Could you check a few things on this model? Use its own coordinates, in mm. Give positions to 0.01 mm unless a question says otherwise; leave off trailing zeros. Order: outer loops, then holes, each group sorted by start corner. A loop starts at its lowest first (then second) coordinate and runs counter-clockwise, first axis right, second up.
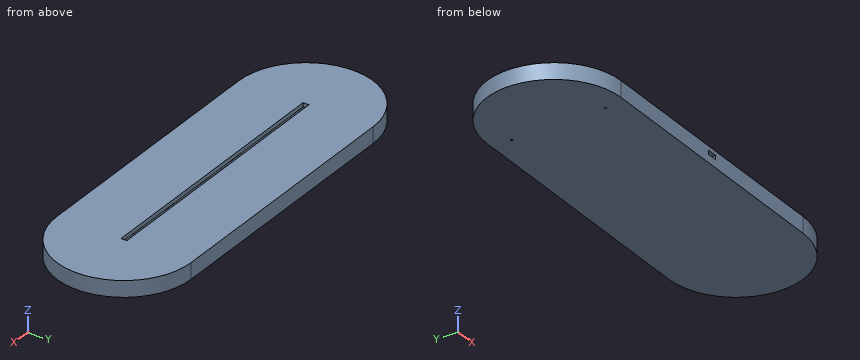
from build123d import *

# Parameters (mm, degrees)
PAD_DEPTH       = 3
PAD001_DEPTH    = 3
SKETCH002_W     = 209.08447
SKETCH002_H     = 4.18
PAD002_DEPTH    = 3
SKETCH003_W     = 26.3
SKETCH003_H     = 34.2
POCKET_DEPTH    = 3
SKETCH004_W     = 18
SKETCH004_H     = 25
POCKET001_DEPTH = 3
SKETCH005_W     = 14
SKETCH005_H     = 5
POCKET002_DEPTH = 6
SKETCH006_W     = 14
SKETCH006_H     = 3
POCKET003_DEPTH = 3
SKETCH007_W     = 8
SKETCH007_H     = 3
POCKET004_DEPTH = 3
SKETCH008_W     = 200
SKETCH008_H     = 4.4
PAD003_DEPTH    = 3
SKETCH009_R     = 0.8
POCKET005_DEPTH = 9


with BuildPart() as part:
    # Sketch → Pad (new body)
    with BuildSketch(Plane.XY):
        with BuildLine():
            ThreePointArc((-100, 50), (-150, 0), (-100, -50))
            Line((-100, -50), (100, -50))
            ThreePointArc((100, -50), (150, 0), (100, 50))
            Line((-100, 50), (100, 50))
        make_face()
    extrude(amount=PAD_DEPTH)

    # Sketch001 (on Face6 of Pad) → Pad001 (join)
    with BuildSketch(Plane.XY.offset(3)):
        with BuildLine():
            ThreePointArc((-100, 50), (-150, 0), (-100, -50))
            Line((-100, -50), (100, -50))
            ThreePointArc((100, -50), (150, 0), (100, 50))
            Line((-100, 50), (100, 50))
        make_face()
        with BuildLine():
            ThreePointArc((-100, 5), (-105, 0), (-100, -5))
            Line((-100, -5), (100, -5))
            ThreePointArc((100, -5), (105, 0), (100, 5))
            Line((-100, 5), (100, 5))
        make_face(mode=Mode.SUBTRACT)
    extrude(amount=PAD001_DEPTH)

    # Sketch002 (on Face9 of Pad001) → Pad002 (join)
    with BuildSketch(Plane.XY.offset(6)):
        with BuildLine():
            ThreePointArc((-100, 50), (-150, 0), (-100, -50))
            Line((-100, -50), (100, -50))
            ThreePointArc((100, -50), (150, 0), (100, 50))
            Line((-100, 50), (100, 50))
        make_face()
        Rectangle(SKETCH002_W, SKETCH002_H, mode=Mode.SUBTRACT)
    extrude(amount=PAD002_DEPTH)

    # Sketch003 (on Face13 of Pad002) → Pocket (cut)
    with BuildSketch(Plane.XY.offset(9)):
        with Locations((0, -29.9)):
            Rectangle(SKETCH003_W, SKETCH003_H)
    extrude(amount=-POCKET_DEPTH, mode=Mode.SUBTRACT)

    # Sketch004 (on Face27 of Pocket) → Pocket001 (cut)
    with BuildSketch(Plane.XY.offset(6)):
        with Locations((0, -25.3)):
            Rectangle(SKETCH004_W, SKETCH004_H)
    extrude(amount=-POCKET001_DEPTH, mode=Mode.SUBTRACT)

    # Sketch005 (on Face13 of Pocket001) → Pocket002 (cut)
    with BuildSketch(Plane.XY.offset(9)):
        with Locations((0, -10.3)):
            Rectangle(SKETCH005_W, SKETCH005_H)
    extrude(amount=-POCKET002_DEPTH, mode=Mode.SUBTRACT)

    # Sketch006 (on Face23 of Pocket002) → Pocket003 (cut)
    with BuildSketch(Plane.XZ.offset(7.8)):
        with Locations((0, 4.5)):
            Rectangle(SKETCH006_W, SKETCH006_H)
    extrude(amount=-POCKET003_DEPTH, mode=Mode.SUBTRACT)

    # Sketch007 (on Face13 of Pocket003) → Pocket004 (cut)
    with BuildSketch(Plane.XY.offset(9)):
        with Locations((0, -48.5)):
            Rectangle(SKETCH007_W, SKETCH007_H)
    extrude(amount=-POCKET004_DEPTH, mode=Mode.SUBTRACT)

    # Sketch008 (on Face15 of Pocket004) → Pad003 (join)
    with BuildSketch(Plane.XY.offset(9)):
        with BuildLine():
            ThreePointArc((-100, 50), (-150, 0), (-100, -50))
            Line((-100, -50), (100, -50))
            ThreePointArc((100, -50), (150, 0), (100, 50))
            Line((-100, 50), (100, 50))
        make_face()
        Rectangle(SKETCH008_W, SKETCH008_H, mode=Mode.SUBTRACT)
    extrude(amount=PAD003_DEPTH)

    # Sketch009 (on Face4 of Pad003) → Pocket005 (cut)
    with BuildSketch(Plane(origin=(0, 0, 0), x_dir=(1, 0, 0), z_dir=(0, 0, -1))):
        with Locations((-95, 35)):
            Circle(SKETCH009_R)
        with Locations((-95, -35)):
            Circle(SKETCH009_R)
    extrude(amount=-POCKET005_DEPTH, mode=Mode.SUBTRACT)


solid = part.part
Item 1: Imagine slicing it at A-A on y = -30.5. List the corners of the cut face in (x, z) for me, then the cut area to 3 significant figures.
Findings:
outline: (-139.62, 0) - (139.62, 0) - (139.62, 12) - (-139.62, 12) - close; hole (-13.15, 6) - (-9, 6) - (-9, 3) - (9, 3) - (9, 6) - (13.15, 6) - (13.15, 9) - (-13.15, 9) - close
area: 3,220 mm2
Item 2: For pin 1 (3 mm diameter, centred on x = -80.5, y = 2.5, fed in from -Z); pin 2 (4 mm diameter, centred on x = -103.5, z = 9, fed in from +Y); pin 3 (3.5 mm diameter, centred on y = -48, z = 8, fed in from +X); pin 4 (1.5 mm diameter, centred on y = -0.5, z = 7.5, fed in from +X), each with a flat end and sliding along its axis, tell me the tip position at first contact or that it passes through.
Findings:
pin 1: stops at z = 0
pin 2: stops at y = 49.98
pin 3: stops at x = 119
pin 4: stops at x = 150
Item 3: Imagine slicing it at B-B on x = -90.5. List the corners of the cut face in (y, z) for me, then the cut area to 3 significant figures.
Findings:
outline: (-50, 0) - (50, 0) - (50, 12) - (2.2, 12) - (2.2, 9) - (2.09, 9) - (2.09, 6) - (5, 6) - (5, 3) - (-5, 3) - (-5, 6) - (-2.09, 6) - (-2.09, 9) - (-2.2, 9) - (-2.2, 12) - (-50, 12) - close
area: 1,140 mm2
Item 4: Imagine slicing it at C-C on x = 127.5. List the corners of the cut face in (y, z) for me, then the cut area to 3 significant figures.
Findings:
outline: (-41.76, 0) - (41.76, 0) - (41.76, 12) - (-41.76, 12) - close
area: 1,000 mm2
Item 5: Please list where these lines run through material, in increasing order: line 1 along Y through (x, z) = (-95, 5); line 2 along Y through (x, z) = (-95, 2); line 3 along Y through (x, z) = (-95, 6.5).
Findings:
line 1: y = -50 to -35.8, -34.2 to -5, 5 to 34.2, 35.8 to 50
line 2: y = -50 to -35.8, -34.2 to 34.2, 35.8 to 50
line 3: y = -50 to -35.8, -34.2 to -2.09, 2.09 to 34.2, 35.8 to 50
